```python
from build123d import *

# Parameters (mm, degrees)
SKETCH1_R           = 4
BOSS_EXTRUDE1_DEPTH = 6.2


with BuildPart() as part:
    # Sketch1 → Boss-Extrude1 (new body)
    with BuildSketch(Plane.XY):
        with BuildLine():
            Line((-16.999999933, -19.000000057), (6.4e-08, -19))
            ThreePointArc((6.4e-08, -19), (18.964168293, -1.166327985), (2.328256926, 18.856808311))
            Line((2.328256926, 18.856808311), (-14.868267557, 20.708519018))
            ThreePointArc((-14.868267557, 20.708519018), (-36.882849209, 1.978880998), (-16.999999933, -19.000000057))
        make_face()
        with Locations(Location((0, 0, 0), (0, 0, 180))):
            Circle(SKETCH1_R, mode=Mode.SUBTRACT)
    extrude(amount=BOSS_EXTRUDE1_DEPTH)


solid = part.part
```
Geometry check sheet. Reference: the model listing, model coordinates, mm. Coordinates: 2 decimals unless noted, no trailing zeros. Write each loop counter-clockwise with the first axis right and the second up, starting at its lowest first coordinate (ties: lowest second). Pieces come first, ordered by that corner, then holes. Notation, with made-up numbers: M 41.25,24 L 80.25,24 A27 cw 80.25,47 Z; hole C 15.25,-8.75 d10. An arc over 180 degrees is marked long. Use one line per item in the form item = value. Start each with the question number.
1) Section check B-B on z = 4. Enter the section's corners in (x, y), and give its area (3 significant figures).
2) Thickness scan on probe 1 along Y at (x, z) = (-1, 2.25); probe 2 along X at (y, z) = (1.5, 4); probe 3 along Y at (x, z) = (-18, 4.5). Record the ranges inside material, lowest first. Write a range as from..to.
3) Section check D-D on y = 7. Enter the section's corners in (x, z), and give its area (3 significant figures).
4) Section check A-A on y = -1. Enter the section's corners in (x, z), and give its area (3 significant figures).
5) Release check for a two-part mould opening along X. For faces 1 (the flat face through (-9, 1, 6.2)), 2 (the cylindrical face through (18.935, -1.567, 3.057)), 3 (the cylindrical face through (0.867, 3.905, 3.057)) record: pulls with the +X half, pulls with the -X half, needs draft (parallel to the pull), parting line crosses it, or undercut.
6) Go/stop test with a flat-tipped pin: pin 1 Ø1.5 at (x, y) = (-27, 10) entering from -Z. Record where the tip stops, or that it passes through.
7) Section check C-C on x = -6. Enter the section's corners in (y, z), and give its area (3 significant figures).
Responses:
q1.outline = M -17,-19 L 0,-19 A19 ccw 2.33,18.86 L -14.87,20.71 A19.91 ccw long Z; hole C 0,0 d8
q1.area = 1,800 mm2
q2.probe_1 = -19..-3.87, 3.87..19.22
q2.probe_2 = -36.9..-3.71, 3.71..18.94
q2.probe_3 = -18.97..20.8
q3.outline = M -35.96,0 L 17.66,0 L 17.66,6.2 L -35.96,6.2 Z
q3.area = 332 mm2
q4.outline = M -36.82,0 L -3.87,0 L -3.87,6.2 L -36.82,6.2 Z; M 3.87,0 L 18.97,0 L 18.97,6.2 L 3.87,6.2 Z
q4.area = 298 mm2
q5.face_1 = needs draft
q5.face_2 = pulls with the +X half
q5.face_3 = undercut
q6.pin_1 = 0
q7.outline = M -19,0 L 19.75,0 L 19.75,6.2 L -19,6.2 Z
q7.area = 240 mm2
